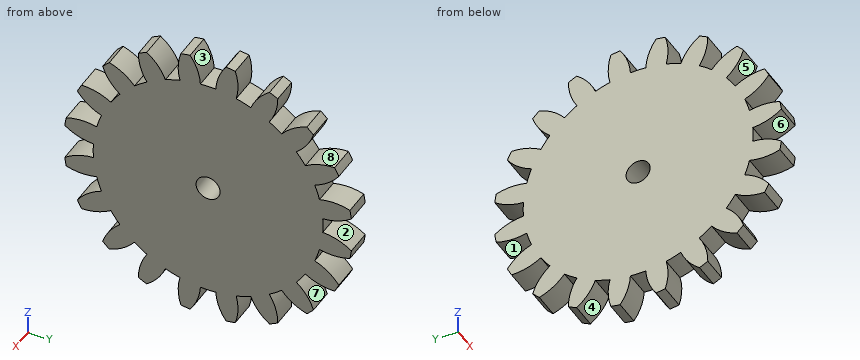
Autodesk Fusion 360 part; units mm, degrees
sketch "Sketch1" plane through (0, 0, 0) normal (1, 0, 0) x (0, 0, -1)
  arc A0 (28.2536, 4.8202) -> (28.2536, 8.3351) centre (2.0635, 6.5776) ccw
  arc A1 (28.2536, 8.3351) -> (34.8066, 10.6867) centre (27.6511, 20.3199) ccw
  arc A2 (17.9851, 35.4827) -> (16.0896, 36.4485) centre (2.0635, 6.5776) ccw
  arc A3 (8.4852, 32.029) -> (8.2737, 38.988) centre (-3.0992, 35.1595) ccw
  arc A4 (34.8066, 10.6867) -> (34.4738, 12.7878) centre (2.0635, 6.5776) ccw
  arc A5 (6.1726, 39.3208) -> (3.8209, 32.7677) centre (15.8058, 32.1653) ccw
  arc A6 (18.8794, -13.5776) -> (24.6337, -17.4969) centre (28.2213, -6.0457) ccw
  arc A7 (16.0896, -23.2932) -> (17.9851, -22.3274) centre (2.0635, 6.5776) ccw
  arc A8 (22.2187, -10.2383) -> (24.2847, -7.3947) centre (2.0635, 6.5776) ccw
  arc A9 (3.8209, 32.7677) -> (0.306, 32.7677) centre (2.0635, 6.5776) ccw
  arc A10 (0.306, -19.6125) -> (3.8209, -19.6125) centre (2.0635, 6.5776) ccw
  arc A11 (24.6337, -17.4969) -> (26.138, -15.9926) centre (2.0635, 6.5776) ccw
  arc A12 (-13.8582, -22.3274) -> (-11.9627, -23.2932) centre (2.0635, 6.5776) ccw
  arc A13 (31.9343, -7.4485) -> (26.4286, -3.187) centre (22.1521, -14.3991) ccw
  arc A14 (6.1726, 39.3208) -> (3.8209, 32.7677) centre (15.8058, 32.1653) ccw
  arc A15 (-14.7525, -13.5776) -> (-11.9089, -15.6436) centre (2.0635, 6.5776) ccw
  arc A16 (8.2737, -25.8327) -> (8.4852, -18.8737) centre (-3.0992, -22.0043) ccw
  arc A17 (-7.7012, -17.7875) -> (-4.3583, -18.8737) centre (2.0635, 6.5776) ccw
  arc A18 (0.306, -19.6125) -> (3.8209, -19.6125) centre (2.0635, 6.5776) ccw
  arc A19 (26.4286, -3.187) -> (27.5148, 0.1559) centre (2.0635, 6.5776) ccw
  arc A20 (8.4852, -18.8737) -> (11.8281, -17.7875) centre (2.0635, 6.5776) ccw
  arc A21 (8.2737, 38.988) -> (6.1726, 39.3208) centre (2.0635, 6.5776) ccw
  arc A22 (6.1726, -26.1655) -> (8.2737, -25.8327) centre (2.0635, 6.5776) ccw
  arc A23 (8.4852, -18.8737) -> (11.8281, -17.7875) centre (2.0635, 6.5776) ccw
  arc A24 (11.8281, -17.7875) -> (16.0896, -23.2932) centre (23.0402, -13.5111) ccw
  arc A25 (30.9685, -9.344) -> (31.9343, -7.4485) centre (2.0635, 6.5776) ccw
  arc A26 (17.9851, -22.3274) -> (16.0358, -15.6436) centre (5.9857, -22.2007) ccw
  arc A27 (6.1726, -26.1655) -> (8.2737, -25.8327) centre (2.0635, 6.5776) ccw
  arc A28 (3.8209, -19.6125) -> (6.1726, -26.1655) centre (15.8058, -19.01) ccw
  arc A29 (34.4738, 0.3674) -> (34.8066, 2.4685) centre (2.0635, 6.5776) ccw
  arc A30 (34.8066, 2.4685) -> (28.2536, 4.8202) centre (27.6511, -7.1647) ccw
  arc A31 (18.8794, 26.7329) -> (16.0358, 28.7989) centre (2.0635, 6.5776) ccw
  arc A32 (-11.9089, -15.6436) -> (-13.8582, -22.3274) centre (-1.8588, -22.2007) ccw
  arc A33 (11.8281, -17.7875) -> (16.0896, -23.2932) centre (23.0402, -13.5111) ccw
  arc A34 (8.4852, 32.029) -> (8.2737, 38.988) centre (-3.0992, 35.1595) ccw
  arc A35 (16.0896, -23.2932) -> (17.9851, -22.3274) centre (2.0635, 6.5776) ccw
  arc A36 (16.0896, 36.4485) -> (11.8281, 30.9428) centre (23.0402, 26.6663) ccw
  arc A37 (16.0358, -15.6436) -> (18.8794, -13.5776) centre (2.0635, 6.5776) ccw
  arc A38 (-4.3583, -18.8737) -> (-4.1467, -25.8327) centre (7.2261, -22.0043) ccw
  arc A39 (-11.9627, -23.2932) -> (-7.7012, -17.7875) centre (-18.9133, -13.5111) ccw
  arc A40 (3.8209, -19.6125) -> (6.1726, -26.1655) centre (15.8058, -19.01) ccw
  arc A41 (11.8281, 30.9428) -> (8.4852, 32.029) centre (2.0635, 6.5776) ccw
  arc A42 (-4.1467, -25.8327) -> (-2.0457, -26.1655) centre (2.0635, 6.5776) ccw
  arc A43 (17.9851, -22.3274) -> (16.0358, -15.6436) centre (5.9857, -22.2007) ccw
  arc A44 (16.0358, -15.6436) -> (18.8794, -13.5776) centre (2.0635, 6.5776) ccw
  arc A45 (24.2847, -7.3947) -> (30.9685, -9.344) centre (30.8418, 2.6554) ccw
  arc A46 (30.9685, 22.4993) -> (24.2847, 20.55) centre (30.8418, 10.4999) ccw
  arc A47 (18.8794, 26.7329) -> (16.0358, 28.7989) centre (2.0635, 6.5776) ccw
  arc A48 (26.138, 29.1479) -> (24.6337, 30.6521) centre (2.0635, 6.5776) ccw
  arc A49 (24.2847, 20.55) -> (22.2187, 23.3936) centre (2.0635, 6.5776) ccw
  arc A50 (27.5148, 12.9994) -> (26.4286, 16.3423) centre (2.0635, 6.5776) ccw
  arc A51 (17.9851, 35.4827) -> (16.0896, 36.4485) centre (2.0635, 6.5776) ccw
  arc A52 (31.9343, 20.6038) -> (30.9685, 22.4993) centre (2.0635, 6.5776) ccw
  arc A53 (8.2737, 38.988) -> (6.1726, 39.3208) centre (2.0635, 6.5776) ccw
  arc A54 (16.0896, 36.4485) -> (11.8281, 30.9428) centre (23.0402, 26.6663) ccw
  arc A55 (24.6337, 30.6521) -> (18.8794, 26.7329) centre (28.2213, 19.201) ccw
  arc A56 (16.0358, 28.7989) -> (17.9851, 35.4827) centre (5.9857, 35.356) ccw
  arc A57 (-2.0457, -26.1655) -> (0.306, -19.6125) centre (-11.6789, -19.01) ccw
  arc A58 (16.0358, 28.7989) -> (17.9851, 35.4827) centre (5.9857, 35.356) ccw
  arc A59 (27.5148, 0.1559) -> (34.4738, 0.3674) centre (30.6454, 11.7403) ccw
  arc A60 (8.2737, -25.8327) -> (8.4852, -18.8737) centre (-3.0992, -22.0043) ccw
  arc A61 (3.8209, 32.7677) -> (0.306, 32.7677) centre (2.0635, 6.5776) ccw
  arc A62 (26.4286, 16.3423) -> (31.9343, 20.6038) centre (22.1521, 27.5544) ccw
  arc A63 (22.2187, 23.3936) -> (26.138, 29.1479) centre (14.6868, 32.7354) ccw
  arc A64 (11.8281, 30.9428) -> (8.4852, 32.029) centre (2.0635, 6.5776) ccw
  arc A65 (34.4738, 12.7878) -> (27.5148, 12.9994) centre (30.6454, 1.4149) ccw
  arc A66 (-27.8074, -7.4485) -> (-26.8416, -9.344) centre (2.0635, 6.5776) ccw
  arc A67 (30.9685, 22.4993) -> (24.2847, 20.55) centre (30.8418, 10.4999) ccw
  arc A68 (-14.7525, -13.5776) -> (-11.9089, -15.6436) centre (2.0635, 6.5776) ccw
  arc A69 (-7.7012, -17.7875) -> (-4.3583, -18.8737) centre (2.0635, 6.5776) ccw
  arc A70 (-4.3583, -18.8737) -> (-4.1467, -25.8327) centre (7.2261, -22.0043) ccw
  arc A71 (-20.5068, -17.4969) -> (-14.7525, -13.5776) centre (-24.0944, -6.0457) ccw
  arc A72 (-13.8582, -22.3274) -> (-11.9627, -23.2932) centre (2.0635, 6.5776) ccw
  arc A73 (-18.0918, -10.2383) -> (-22.0111, -15.9926) centre (-10.5599, -19.5802) ccw
  arc A74 (-30.6797, 2.4685) -> (-30.3469, 0.3674) centre (2.0635, 6.5776) ccw
  arc A75 (-27.8074, 20.6038) -> (-22.3017, 16.3423) centre (-18.0252, 27.5544) ccw
  arc A76 (-11.9089, 28.7989) -> (-14.7525, 26.7329) centre (2.0635, 6.5776) ccw
  arc A77 (24.6337, 30.6521) -> (18.8794, 26.7329) centre (28.2213, 19.201) ccw
  arc A78 (-18.0918, 23.3936) -> (-20.1578, 20.55) centre (2.0635, 6.5776) ccw
  arc A79 (-30.3469, 0.3674) -> (-23.3879, 0.1559) centre (-26.5185, 11.7403) ccw
  arc A80 (34.4738, 0.3674) -> (34.8066, 2.4685) centre (2.0635, 6.5776) ccw
  arc A81 (-7.7012, 30.9428) -> (-11.9627, 36.4485) centre (-18.9133, 26.6663) ccw
  arc A82 (34.8066, 2.4685) -> (28.2536, 4.8202) centre (27.6511, -7.1647) ccw
  arc A83 (-4.1467, 38.988) -> (-4.3583, 32.029) centre (7.2261, 35.1595) ccw
  arc A84 (-18.0918, -10.2383) -> (-22.0111, -15.9926) centre (-10.5599, -19.5802) ccw
  arc A85 (26.138, 29.1479) -> (24.6337, 30.6521) centre (2.0635, 6.5776) ccw
  arc A86 (-22.0111, -15.9926) -> (-20.5068, -17.4969) centre (2.0635, 6.5776) ccw
  arc A87 (-20.1578, -7.3947) -> (-18.0918, -10.2383) centre (2.0635, 6.5776) ccw
  arc A88 (-24.1266, 8.3351) -> (-24.1266, 4.8202) centre (2.0635, 6.5776) ccw
  arc A89 (-26.8416, -9.344) -> (-20.1578, -7.3947) centre (-26.7149, 2.6554) ccw
  arc A90 (22.2187, 23.3936) -> (26.138, 29.1479) centre (14.6868, 32.7354) ccw
  arc A91 (28.2536, 4.8202) -> (28.2536, 8.3351) centre (2.0635, 6.5776) ccw
  arc A92 (24.6337, -17.4969) -> (26.138, -15.9926) centre (2.0635, 6.5776) ccw
  arc A93 (-27.8074, -7.4485) -> (-26.8416, -9.344) centre (2.0635, 6.5776) ccw
  arc A94 (22.2187, -10.2383) -> (24.2847, -7.3947) centre (2.0635, 6.5776) ccw
  arc A95 (34.8066, 10.6867) -> (34.4738, 12.7878) centre (2.0635, 6.5776) ccw
  arc A96 (27.5148, 12.9994) -> (26.4286, 16.3423) centre (2.0635, 6.5776) ccw
  arc A97 (24.2847, 20.55) -> (22.2187, 23.3936) centre (2.0635, 6.5776) ccw
  arc A98 (28.2536, 8.3351) -> (34.8066, 10.6867) centre (27.6511, 20.3199) ccw
  arc A99 (-26.8416, 22.4993) -> (-27.8074, 20.6038) centre (2.0635, 6.5776) ccw
  arc A100 (-11.9627, -23.2932) -> (-7.7012, -17.7875) centre (-18.9133, -13.5111) ccw
  arc A101 (27.5148, 0.1559) -> (34.4738, 0.3674) centre (30.6454, 11.7403) ccw
  arc A102 (34.4738, 12.7878) -> (27.5148, 12.9994) centre (30.6454, 1.4149) ccw
  arc A103 (-22.3017, -3.187) -> (-27.8074, -7.4485) centre (-18.0252, -14.3991) ccw
  arc A104 (-20.5068, 30.6521) -> (-22.0111, 29.1479) centre (2.0635, 6.5776) ccw
  arc A105 (26.138, -15.9926) -> (22.2187, -10.2383) centre (14.6868, -19.5802) ccw
  arc A106 (26.4286, -3.187) -> (27.5148, 0.1559) centre (2.0635, 6.5776) ccw
  arc A107 (18.8794, -13.5776) -> (24.6337, -17.4969) centre (28.2213, -6.0457) ccw
  arc A108 (30.9685, -9.344) -> (31.9343, -7.4485) centre (2.0635, 6.5776) ccw
  arc A109 (31.9343, -7.4485) -> (26.4286, -3.187) centre (22.1521, -14.3991) ccw
  arc A110 (-23.3879, 0.1559) -> (-22.3017, -3.187) centre (2.0635, 6.5776) ccw
  arc A111 (26.4286, 16.3423) -> (31.9343, 20.6038) centre (22.1521, 27.5544) ccw
  arc A112 (31.9343, 20.6038) -> (30.9685, 22.4993) centre (2.0635, 6.5776) ccw
  arc A113 (-30.3469, 0.3674) -> (-23.3879, 0.1559) centre (-26.5185, 11.7403) ccw
  arc A114 (24.2847, -7.3947) -> (30.9685, -9.344) centre (30.8418, 2.6554) ccw
  arc A115 (-14.7525, 26.7329) -> (-20.5068, 30.6521) centre (-24.0944, 19.201) ccw
  arc A116 (-26.8416, -9.344) -> (-20.1578, -7.3947) centre (-26.7149, 2.6554) ccw
  arc A117 (-20.1578, -7.3947) -> (-18.0918, -10.2383) centre (2.0635, 6.5776) ccw
  arc A118 (0.306, 32.7677) -> (-2.0457, 39.3208) centre (-11.6789, 32.1653) ccw
  arc A119 (-24.1266, 4.8202) -> (-30.6797, 2.4685) centre (-23.5242, -7.1647) ccw
  arc A120 (-26.8416, 22.4993) -> (-27.8074, 20.6038) centre (2.0635, 6.5776) ccw
  arc A121 (-30.3469, 12.7878) -> (-30.6797, 10.6867) centre (2.0635, 6.5776) ccw
  arc A122 (-11.9089, -15.6436) -> (-13.8582, -22.3274) centre (-1.8588, -22.2007) ccw
  arc A123 (-4.1467, -25.8327) -> (-2.0457, -26.1655) centre (2.0635, 6.5776) ccw
  arc A124 (-23.3879, 12.9994) -> (-30.3469, 12.7878) centre (-26.5185, 1.4149) ccw
  arc A125 (-22.0111, 29.1479) -> (-18.0918, 23.3936) centre (-10.5599, 32.7354) ccw
  arc A126 (-22.3017, -3.187) -> (-27.8074, -7.4485) centre (-18.0252, -14.3991) ccw
  arc A127 (-20.5068, -17.4969) -> (-14.7525, -13.5776) centre (-24.0944, -6.0457) ccw
  arc A128 (-4.3583, 32.029) -> (-7.7012, 30.9428) centre (2.0635, 6.5776) ccw
  arc A129 (-2.0457, 39.3208) -> (-4.1467, 38.988) centre (2.0635, 6.5776) ccw
  arc A130 (-18.0918, 23.3936) -> (-20.1578, 20.55) centre (2.0635, 6.5776) ccw
  arc A131 (-23.3879, 0.1559) -> (-22.3017, -3.187) centre (2.0635, 6.5776) ccw
  arc A132 (-20.1578, 20.55) -> (-26.8416, 22.4993) centre (-26.7149, 10.4999) ccw
  arc A133 (-27.8074, 20.6038) -> (-22.3017, 16.3423) centre (-18.0252, 27.5544) ccw
  arc A134 (-2.0457, -26.1655) -> (0.306, -19.6125) centre (-11.6789, -19.01) ccw
  arc A135 (-22.0111, -15.9926) -> (-20.5068, -17.4969) centre (2.0635, 6.5776) ccw
  arc A136 (-24.1266, 8.3351) -> (-24.1266, 4.8202) centre (2.0635, 6.5776) ccw
  arc A137 (-24.1266, 4.8202) -> (-30.6797, 2.4685) centre (-23.5242, -7.1647) ccw
  arc A138 (-14.7525, 26.7329) -> (-20.5068, 30.6521) centre (-24.0944, 19.201) ccw
  arc A139 (-11.9627, 36.4485) -> (-13.8582, 35.4827) centre (2.0635, 6.5776) ccw
  arc A140 (-2.0457, 39.3208) -> (-4.1467, 38.988) centre (2.0635, 6.5776) ccw
  arc A141 (-20.1578, 20.55) -> (-26.8416, 22.4993) centre (-26.7149, 10.4999) ccw
  arc A142 (-30.3469, 12.7878) -> (-30.6797, 10.6867) centre (2.0635, 6.5776) ccw
  arc A143 (-20.5068, 30.6521) -> (-22.0111, 29.1479) centre (2.0635, 6.5776) ccw
  arc A144 (-4.1467, 38.988) -> (-4.3583, 32.029) centre (7.2261, 35.1595) ccw
  arc A145 (-11.9627, 36.4485) -> (-13.8582, 35.4827) centre (2.0635, 6.5776) ccw
  arc A146 (-30.6797, 2.4685) -> (-30.3469, 0.3674) centre (2.0635, 6.5776) ccw
  arc A147 (0.306, 32.7677) -> (-2.0457, 39.3208) centre (-11.6789, 32.1653) ccw
  arc A148 (-23.3879, 12.9994) -> (-30.3469, 12.7878) centre (-26.5185, 1.4149) ccw
  arc A149 (-13.8582, 35.4827) -> (-11.9089, 28.7989) centre (-1.8588, 35.356) ccw
  arc A150 (-13.8582, 35.4827) -> (-11.9089, 28.7989) centre (-1.8588, 35.356) ccw
  arc A151 (-22.3017, 16.3423) -> (-23.3879, 12.9994) centre (2.0635, 6.5776) ccw
  arc A152 (-4.3583, 32.029) -> (-7.7012, 30.9428) centre (2.0635, 6.5776) ccw
  arc A153 (-11.9089, 28.7989) -> (-14.7525, 26.7329) centre (2.0635, 6.5776) ccw
  arc A154 (-22.3017, 16.3423) -> (-23.3879, 12.9994) centre (2.0635, 6.5776) ccw
  arc A155 (-22.0111, 29.1479) -> (-18.0918, 23.3936) centre (-10.5599, 32.7354) ccw
  arc A156 (-7.7012, 30.9428) -> (-11.9627, 36.4485) centre (-18.9133, 26.6663) ccw
  arc A157 (-30.6797, 10.6867) -> (-24.1266, 8.3351) centre (-23.5242, 20.3199) ccw
  arc A158 (-30.6797, 10.6867) -> (-24.1266, 8.3351) centre (-23.5242, 20.3199) ccw
  arc A159 (26.138, -15.9926) -> (22.2187, -10.2383) centre (14.6868, -19.5802) ccw
  circle A160 centre (2.0635, 6.5776) radius 2.75
  dimension "d4" = 5.5
extrude "Extrude1" add sketch "Sketch1" along normal blind 6
Work out the finished part from the listing and answer in its coordinate system (mm). Face numbers are marked on the shaded views. A direction names the side the tool comes from. Give positions to 0.01 mm unless a question says otherwise; leave off trailing zeros. Loops run counter-clockwise (first coordinate to the right, second up) from the corner with the lowest first, then second, coordinate; pieces in that order, holes last. Notation, with made-up numbers: (14, 81.5) -> (49, 81.5) arc R20 ccw to (49, 88.5) -> close; hole circle Ø4 at (89, -31.5). An arc over 180 degrees is marked (long way). One line per question, with ' | ' between items. Start each with the question number.
1) Section B-B, the plane y = -2 is taken. Determine the outline of the cut face in (x, z), then the cut area to 3 significant figures.
2) For the marked faces 1, 2, 3, 4 and 5, determine the directions among +Z, -Z, +X, -X, +Y, -Y from which every point of the face is accessible in a straight line to the end or side of a thin tool.
3) This flat-tipped pin is pushed along its axis until it touches: pin 1 (3 mm diameter, centred on x = 3.5, y = -2.5, fed in from +Z). Where does it stop, or does it pass through?
4) Straight lines are drawn through the part: L1, parallel to Z at x = 2.9, y = 6.5; L2, parallel to Z at x = 2.85, y = 27.5; L3, parallel to Z at x = 4.65, y = 30. For each, find the intervals that lie inside material, in ascending order.
5) Determine the mould class of the marked faces 6, 7 and 8 for opening direction Y: +Y half, -Y half, draft (parallel to the pull), parting line (faces both ways), or undercut.
6) Section A-A, the plane z = -14 is taken. Determine the outline of the cut face in (x, y), then the cut area to 3 significant figures.
Resolved:
1) outline: (0, -26.87) -> (6, -26.87) -> (6, 22.74) -> (0, 22.74) -> close | area: 298 mm2
2) face 1: +X, -X | face 2: +X, -X, +Y | face 3: +Z, +X, -X | face 4: -Z, +X, -X | face 5: +X, -X, -Y
3) pin 1: z = 24.01
4) L1: -28.31 to -4.81, 0.69 to 24.19 | L2: -25.48 to -19.55, -17.91 to 13.79, 15.43 to 21.36 | L3: -25.31 to -22.99, -16.72 to 12.6, 18.86 to 21.18
5) face 6: -Y half | face 7: +Y half | face 8: undercut
6) outline: (0, -21.4) -> (6, -21.4) -> (6, 34.56) -> (0, 34.56) -> close | area: 336 mm2
